```python
from build123d import *

# Parameters (mm, degrees)
BOSS_EXTRUDE1_DEPTH   = 80
CORTE_EXTRUS_O1_DEPTH = 10
SKETCH3_W             = 5
SKETCH3_H             = 80
BOSS_EXTRUDE2_DEPTH   = 50
SKETCH4_W             = 80
SKETCH4_H             = 9.86245083
BOSS_EXTRUDE3_DEPTH   = 100
SKETCH5_R             = 1.5
CUT_EXTRUDE1_DEPTH    = 40
SKETCH6_W             = 5
SKETCH6_H             = 80
BOSS_EXTRUDE4_DEPTH   = 40
SKETCH7_R             = 1.5
CUT_EXTRUDE2_DEPTH    = 40
SKETCH8_W             = 80
SKETCH8_H             = 10
BOSS_EXTRUDE5_DEPTH   = 40
SKETCH9_R             = 1.5
SKETCH9_R_2           = 17.5
CUT_EXTRUDE3_DEPTH    = 40


with BuildPart() as part:
    # Sketch1 → Boss-Extrude1 (new body)
    with BuildSketch(Plane.XY):
        Polygon((0, 0), (0, 30), (12.8, 30), (12.8, 0), (7.8, 0), (7.8, 10), (6, 10), (6, 0), align=None)
    extrude(amount=BOSS_EXTRUDE1_DEPTH)

    # Esboço2 → Corte-extrusão1 (cut)
    with BuildSketch(Plane.XZ):
        with BuildLine():
            Line((6, 80), (6, 0))
            ThreePointArc((6, 0), (-2.670710227, 40), (6, 80))
        make_face()
    extrude(amount=-CORTE_EXTRUS_O1_DEPTH, mode=Mode.SUBTRACT)

    # Sketch3 → Boss-Extrude2 (add)
    with BuildSketch(Plane.XZ):
        with Locations((10.3, 40)):
            Rectangle(SKETCH3_W, SKETCH3_H)
    extrude(amount=BOSS_EXTRUDE2_DEPTH)

    # Sketch4 → Boss-Extrude3 (add)
    with BuildSketch(Plane.ZY):
        with Locations((40, 4.931225415)):
            Rectangle(SKETCH4_W, SKETCH4_H)
    extrude(amount=BOSS_EXTRUDE3_DEPTH)

    # Sketch5 → Cut-Extrude1 (cut)
    with BuildSketch(Plane(origin=(0, 9.86245083, 0), x_dir=(1, 0, 0), z_dir=(0, 1, 0))):
        with Locations(Location((-6.5, -21.55, 0), (0, 0, 270))):
            Circle(SKETCH5_R)
        with Locations(Location((-6.5, -58.45, 0), (0, 0, 270))):
            Circle(SKETCH5_R)
        with Locations(Location((-43.4, -21.55, 0), (0, 0, 270))):
            Circle(SKETCH5_R)
        with Locations(Location((-43.4, -58.45, 0), (0, 0, 270))):
            Circle(SKETCH5_R)
        with Locations(Location((-55.6, -64.85, 0), (0, 0, 270))):
            Circle(SKETCH5_R)
        with Locations(Location((-95, -64.85, 0), (0, 0, 270))):
            Circle(SKETCH5_R)
        with Locations(Location((-95, -15.15, 0), (0, 0, 270))):
            Circle(SKETCH5_R)
    extrude(amount=-CUT_EXTRUDE1_DEPTH, mode=Mode.SUBTRACT)

    # Sketch6 → Boss-Extrude4 (add)
    with BuildSketch(Plane(origin=(0, 30, 0), x_dir=(1, 0, 0), z_dir=(0, 1, 0))):
        with Locations((10.3, -40)):
            Rectangle(SKETCH6_W, SKETCH6_H)
    extrude(amount=BOSS_EXTRUDE4_DEPTH)

    # Sketch7 → Cut-Extrude2 (cut)
    with BuildSketch(Plane(origin=(12.8, 0, 0), x_dir=(0, 0, -1), z_dir=(1, 0, 0))):
        with Locations(Location((-77.5, 66, 0), (0, 0, 90))):
            Circle(SKETCH7_R)
        with Locations(Location((-2.5, 66, 0), (0, 0, 90))):
            Circle(SKETCH7_R)
        with Locations(Location((-2.5, 34.7, 0), (0, 0, 90))):
            Circle(SKETCH7_R)
        with Locations(Location((-77.5, 34.7, 0), (0, 0, 90))):
            Circle(SKETCH7_R)
        Polygon((-74, 68.5), (-74, 62), (-76, 62), (-76, 37.5), (0, 37.5), (0, 62), (-34, 62), (-34, 68.5), align=None)
    extrude(amount=-CUT_EXTRUDE2_DEPTH, mode=Mode.SUBTRACT)

    # Sketch8 → Boss-Extrude5 (add)
    with BuildSketch(Plane(origin=(12.8, 0, 0), x_dir=(0, 0, -1), z_dir=(1, 0, 0))):
        with Locations((-40, 5)):
            Rectangle(SKETCH8_W, SKETCH8_H)
    extrude(amount=BOSS_EXTRUDE5_DEPTH)

    # Sketch9 → Cut-Extrude3 (cut)
    with BuildSketch(Plane(origin=(0, 10, 0), x_dir=(1, 0, 0), z_dir=(0, 1, 0))):
        with Locations(Location((47.8, -65, 0), (0, 0, 180))):
            Circle(SKETCH9_R)
        with Locations(Location((17.8, -65, 0), (0, 0, 180))):
            Circle(SKETCH9_R)
        with Locations(Location((47.8, -15, 0), (0, 0, 180))):
            Circle(SKETCH9_R)
        with Locations(Location((17.8, -15, 0), (0, 0, 180))):
            Circle(SKETCH9_R)
        with Locations(Location((33.099545745, -40, 0), (0, 0, 180))):
            Circle(SKETCH9_R_2)
    extrude(amount=-CUT_EXTRUDE3_DEPTH, mode=Mode.SUBTRACT)


solid = part.part
```
Read the model definition and answer for the solid it produces. Units are mm, in the model's axes. A direction names the side the tool comes from. Coordinates: 2 decimals unless noted, no trailing zeros. Loops run counter-clockwise (first coordinate to the right, second up) from the corner with the lowest first, then second, coordinate; pieces in that order, holes last.
(1) The mould has two halves that part along Y. Classify faces 5 (the face through (4, 30, 39)), 6 (the face through (12.8, 26, 41)), 7 (the face through (10, 65, 74)), 8 (the face through (10, 50, 76)): released by +Y, released by -Y, zero draft, split by the parting line, or undercut.
Solution:
face 5: released by +Y
face 6: zero draft
face 7: undercut
face 8: undercut
(2) Consider line 1 along X through (y, z) = (2.5, 58.45); line 2 along Z through (x, y) = (10, 66); line 3 along Z through (x, y) = (9.1, 34.7). Determine where each line is inside the solid, lowest interval first.
Solution:
line 1: x = -100 to -44.9, -41.9 to -8, -5 to 0, 7.8 to 52.8
line 2: z = 0 to 1, 4 to 34, 74 to 76, 79 to 80
line 3: z = 0 to 1, 4 to 76, 79 to 80
(3) The part is cut by section B-B (z = 38). Determine the outline of the cut face in (x, y), and give its area (3 significant figures).
Solution:
outline: (-100, 0) - (0, 0) - (0, 9.86) - (-100, 9.86) - close; (0, 10) - (7.8, 10) - (7.8, -50) - (12.8, -50) - (12.8, 0) - (15.71, 0) - (15.71, 10) - (12.8, 10) - (12.8, 37.5) - (7.8, 37.5) - (7.8, 30) - (0, 30) - close; (7.8, 68.5) - (12.8, 68.5) - (12.8, 70) - (7.8, 70) - close; (50.48, 0) - (52.8, 0) - (52.8, 10) - (50.48, 10) - close
area: 1,640 mm2
(4) The part is cut by section C-C (x = 31.5). Determine the outline of the cut face in (y, z), and give its area (3 significant figures).
Solution:
outline: (0, 0) - (10, 0) - (10, 22.57) - (0, 22.57) - close; (0, 57.43) - (10, 57.43) - (10, 80) - (0, 80) - close
area: 451 mm2
(5) A tool of negligible diameter and unlimited length cuts with its end or side. For faces 1 (the face through (7.8, -20, 39)), 2 (the face through (7.8, 36, 41)), 3 (the face through (2.625, 4.93, 8.455)), 4 (the face through (10, 62, 17)), from which of +Z, -Z, +X, -X, +Y, -Y can it reach the whole face along a straight path? Write none if from no direction.
Solution:
face 1: +Z, -Z, -Y
face 2: +Z, -Z, -X, +Y
face 3: -Y
face 4: -Z, +X, -X
(6) Flat-ended cylindrical pins translate along their axes: pin 1 Ø4 at (x, z) = (17.8, 65) entering from -Y; pin 2 Ø6 at (x, z) = (16.5, 61) entering from +Y; pin 3 Ø1.8 at (x, z) = (-95, 64.85) entering from +Y; pin 4 Ø3 at (x, z) = (-70.5, 54) entering from +Y. Find the tip coordinate at first contact, or state that the pin passes through.
Solution:
pin 1: stops at y = 0
pin 2: stops at y = 10
pin 3: passes through
pin 4: stops at y = 9.86
(7) The part is cut by section D-D (z = 6). Determine the outline of the cut face in (x, y), and give its area (3 significant figures).
Solution:
outline: (-100, 0) - (3.51, 0) - (3.51, 10) - (7.8, 10) - (7.8, -50) - (12.8, -50) - (12.8, 0) - (52.8, 0) - (52.8, 10) - (12.8, 10) - (12.8, 37.5) - (7.8, 37.5) - (7.8, 30) - (0, 30) - (0, 9.86) - (-100, 9.86) - close; (7.8, 62) - (12.8, 62) - (12.8, 70) - (7.8, 70) - close
area: 2,050 mm2
(8) The part is cut by section A-A (y = 5). Count the separate pieces of the cut face and the enclosed holes in it, and give its area (3 significant figures).
Solution:
separate pieces: 2
enclosed holes: 12
area: 10,700 mm2
